```python
from build123d import *

# Parameters (mm, degrees)
SKIZZE1_W                       = 247.6
SKIZZE1_H                       = 178.5
AUFSATZ_LINEAR_AUSTRAGEN1_DEPTH = 6.1
VERRUNDUNG1_R                   = 12
SKIZZE2_R                       = 6
AUFSATZ_LINEAR_AUSTRAGEN2_DEPTH = 2
VERRUNDUNG2_R                   = 1.5
AUFSATZ_LINEAR_AUSTRAGEN3_DEPTH = 0.5
AUFSATZ_LINEAR_AUSTRAGEN5_DEPTH = 0.5


with BuildPart() as part:
    # Skizze1 → Aufsatz-Linear austragen1 (new body)
    with BuildSketch(Plane(origin=(0, 0, 0), x_dir=(1, 0, 0), z_dir=(0, 1, 0))):
        Rectangle(SKIZZE1_W, SKIZZE1_H)
    extrude(amount=AUFSATZ_LINEAR_AUSTRAGEN1_DEPTH)

    # Verrundung1
    verrundung1_edges = [part.edges().sort_by_distance(p)[0] for p in [
        (-123.8, 3.05, -89.25),
        (123.8, 3.05, -89.25),
        (123.8, 3.05, 89.25),
        (-123.8, 3.05, 89.25),
    ]]
    fillet(verrundung1_edges, radius=VERRUNDUNG1_R)

    # Skizze2 → Aufsatz-Linear austragen2 (add)
    with BuildSketch(Plane(origin=(0, 6.1, 0), x_dir=(1, 0, 0), z_dir=(0, 1, 0))):
        with Locations((-111.8, -77.25)):
            Circle(SKIZZE2_R)
    extrude(amount=AUFSATZ_LINEAR_AUSTRAGEN2_DEPTH)

    # Verrundung2
    verrundung2_edges = [part.edges().sort_by_distance(p)[0] for p in [
        (-117.8, 6.1, 77.25),
    ]]
    fillet(verrundung2_edges, radius=VERRUNDUNG2_R)

    # Skizze3 → Aufsatz-Linear austragen3 (add)
    with BuildSketch(Plane.ZY.offset(123.8)):
        with BuildLine():
            Line((74.4, 1.2), (61.1, 1.2))
            ThreePointArc((61.1, 1.2), (59.25, 3.05), (61.1, 4.9))
            Line((61.1, 4.9), (74.4, 4.9))
            ThreePointArc((74.4, 4.9), (76.25, 3.05), (74.4, 1.2))
        make_face()
    extrude(amount=AUFSATZ_LINEAR_AUSTRAGEN3_DEPTH)

    # Skizze4 → Aufsatz-Linear austragen5 (add)
    with BuildSketch(Plane.XY.offset(89.25)):
        with BuildLine():
            Line((-102.8, 4.05), (-94.8, 4.05))
            ThreePointArc((-94.8, 4.05), (-93.8, 3.05), (-94.8, 2.05))
            Line((-94.8, 2.05), (-102.8, 2.05))
            ThreePointArc((-102.8, 2.05), (-103.8, 3.05), (-102.8, 4.05))
        make_face()
        with BuildLine():
            Line((-90.8, 4.05), (-82.8, 4.05))
            ThreePointArc((-82.8, 4.05), (-81.8, 3.05), (-82.8, 2.05))
            Line((-82.8, 2.05), (-90.8, 2.05))
            ThreePointArc((-90.8, 2.05), (-91.8, 3.05), (-90.8, 4.05))
        make_face()
    extrude(amount=AUFSATZ_LINEAR_AUSTRAGEN5_DEPTH)


solid = part.part
```
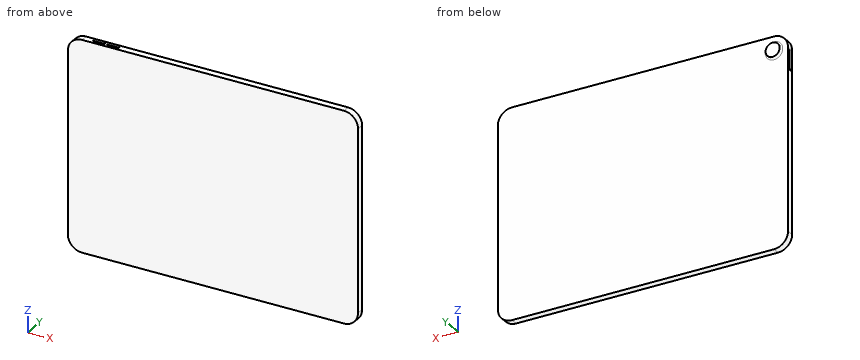
The listing builds one solid part. Answer for the finished solid, in the listing's coordinates (mm). Coordinates: 2 decimals unless noted, no trailing zeros. Write each loop counter-clockwise with the first axis right and the second up, starting at its lowest first coordinate (ties: lowest second). Pieces come first, ordered by that corner, then holes. Notation, with made-up numbers: (46, 89.5) - (82, 89.5) arc R20 ccw to (82, 106.5) - close; hole circle Ø3 at (-3.75, -6.75). An arc over 180 degrees is marked (long way). Return JSON: item names as keys, results as strings. Group by question number.
Q1. The part is cut by section A-A on z = -24. Write down the section's boundary in (x, y).
Q2. The part is cut by section B-B on x = -52. Write down the section's boundary in (y, z).
Q3. Flat-ended cylindrical pins translate along their axes: pin 1 Ø4 at (x, z) = (78.5, -51.5) entering from +Y; pin 2 Ø1.8 at (y, z) = (2, 3) entering from -X; pin 3 Ø3 at (x, y) = (-10, 2) entering from +Z. Find the tip coordinate at first contact, or state that the pin passes through.
Q4. Find the intervals of material crossed by line 1 along Z through (x, y) = (96, 3); line 2 along Y through (x, z) = (9.5, -71); line 3 along X through (y, z) = (2.75, -69.5), in increasing order. Write a range as [from, to].
Evaluation:
{
 "1": {"outline": "(-123.8, 0) - (123.8, 0) - (123.8, 6.1) - (-123.8, 6.1) - close"},
 "2": {"outline": "(0, -89.25) - (6.1, -89.25) - (6.1, 89.25) - (0, 89.25) - close"},
 "3": {"pin 1": "stops at y = 6.1", "pin 2": "stops at x = -123.8", "pin 3": "stops at z = 89.25"},
 "4": {"line 1": "z = [-89.25, 89.25]", "line 2": "y = [0, 6.1]", "line 3": "x = [-123.8, 123.8]"}
}
